```python
from build123d import *

# Parameters (mm, degrees)
BOSS_EXTRUDE1_DEPTH = 20
SKETCH3_R           = 1.5
CUT_EXTRUDE1_DEPTH  = 10
FILLET1_R           = 1.5


with BuildPart() as part:
    # Sketch2 → Boss-Extrude1 (new body)
    with BuildSketch(Plane.XY):
        with BuildLine():
            Line((-148, -28), (-153, -28))
            ThreePointArc((-153, -28), (-154.414213562, -28.585786438), (-155, -30))
            Line((-155, -30), (-155, -66))
            ThreePointArc((-155, -66), (-154.414213562, -67.414213562), (-153, -68))
            Line((-153, -68), (-148, -68))
            Line((-148, -68), (-148, -28))
        make_face()
    extrude(amount=BOSS_EXTRUDE1_DEPTH)

    # Sketch3 → Cut-Extrude1 (cut)
    with BuildSketch(Plane(origin=(-148, 0, 0), x_dir=(0, 0, -1), z_dir=(1, 0, 0))):
        with Locations((-15, -63.625)):
            Circle(SKETCH3_R)
        with Locations((-5, -32.375)):
            Circle(SKETCH3_R)
        with Locations((-15, -32.375)):
            Circle(SKETCH3_R)
    extrude(amount=-CUT_EXTRUDE1_DEPTH, mode=Mode.SUBTRACT)

    # Fillet1
    fillet1_edges = [part.edges().sort_by_distance(p)[0] for p in [
        (-150.5, -68, 20),
        (-150.5, -28, 20),
        (-154.414213562, -28.585786438, 20),
        (-155, -48, 20),
        (-154.414213562, -67.414213562, 20),
    ]]
    fillet(fillet1_edges, radius=FILLET1_R)


solid = part.part
```
Here's how the part is built. I have some questions about the finished solid (model axes, mm). Round coordinates to 2 decimals unless told otherwise and drop trailing zeros. Write each loop counter-clockwise with the first axis right and the second up, starting at its lowest first coordinate (ties: lowest second). Pieces come first, ordered by that corner, then holes. Notation, with made-up numbers: M 24,70.25 L 66,70.25 A9 cw 66,87.25 Z; hole C -21,-34.5 d8. An arc over 180 degrees is marked long. Answer as CSV lines item,"result". Start each with the question number.
1. Thinking about a two-plate mould opening in Z: for faces 1 (the cylindrical face through (-154.55, -48.25, 19.57)), 2 (the cylindrical face through (-151.451, -62.611, 16.106)), 3 (the flat face through (-151, -68, 9)), 4 (the cylindrical face through (-151.45, -33.84, 5.33)), which applies, released by +Z, released by -Z, zero draft, split by the parting line, or undercut?
2. Suppose I cut it at D-D on x = -151.25. Write out the boundary of the cut face in (y, z) (3 decimals).
3. Suppose I cut it at B-B on y = -33.5. Write out the boundary of the cut face in (x, z).
4. Suppose I cut it at A-A on z = 15. Write out the boundary of the cut face in (x, y) (3 decimals).
5. Suppose I cut it at C-C on z = 5. Write out the boundary of the cut face in (x, y) (3 decimals), then the cut area to 3 significant figures.
6. I need wall thicknesses on probe 1 along Y at (x, z) = (-151.25, 15) (3 decimals); probe 2 along Y at (x, z) = (-154, 15) (3 decimals); probe 3 along Z at (x, y) = (-153, -32). Which ranges of each line are inside material? Lowest first, please.
Check result:
1,face 1,"released by +Z"
1,face 2,"undercut"
1,face 3,"zero draft"
1,face 4,"undercut"
2,outline,"M -68,0 L -28,0 L -28,18.5 A1.5 ccw -29.5,20 L -66.5,20 A1.5 ccw -68,18.5 Z; hole C -63.625,15 d3; hole C -32.375,5 d3; hole C -32.375,15 d3"
3,outline,"M -155,0 L -148,0 L -148,4.01 L -155,4.01 Z; M -155,5.99 L -148,5.99 L -148,14.01 L -155,14.01 Z; M -155,15.99 L -148,15.99 L -148,20 L -153.5,20 A1.5 ccw -155,18.5 Z"
4,outline,"M -155,-66 A2 ccw -153,-68 L -148,-68 L -148,-65.125 L -155,-65.125 Z; M -155,-62.125 L -148,-62.125 L -148,-33.875 L -155,-33.875 Z; M -155,-30.875 L -148,-30.875 L -148,-28 L -153,-28 A2 ccw -155,-30 Z"
5,outline,"M -155,-66 A2 ccw -153,-68 L -148,-68 L -148,-33.875 L -155,-33.875 Z; M -155,-30.875 L -148,-30.875 L -148,-28 L -153,-28 A2 ccw -155,-30 Z"
5,area,"257 mm2"
6,probe 1,"y = -68 to -65.125, -62.125 to -33.875, -30.875 to -28"
6,probe 2,"y = -67.732 to -65.125, -62.125 to -33.875, -30.875 to -28.268"
6,probe 3,"z = 0 to 3.55, 6.45 to 13.55, 16.45 to 20"
